Check sheet for the modelled part. Datum: model origin and axes. Units: mm. A direction names the side the tool comes from. Give positions to 0.01 mm unless a question says otherwise; leave off trailing zeros. Write each loop counter-clockwise with the first axis right and the second up, starting at its lowest first coordinate (ties: lowest second). Pieces come first, ordered by that corner, then holes. Notation, with made-up numbers: M -37.75,52.25 L -6.75,52.25 A25 ccw -6.75,83.25 Z; hole C 20.25,58.25 d3. An arc over 180 degrees is marked long. Write item = value, one per line. Start each with the question number.
1) Cross-section at A-A, the plane z = 12.5. Record the cut outline in (x, y).
2) Go/stop test with a flat-tipped pin: pin 1 (4 mm diameter, centred on x = -49.5, y = 2, fed in from +Z). Record where the tip stops, or that it passes through.
3) Mould release check, pull along Y, two halves, no side actions. Record for faces 1 (the flat face through (63.5, 5, 16)), 2 (the flat face through (-53.1, 15, 20.5)), 3 (the flat face through (-1, -25.4, 16)): released by +Y, released by -Y, zero draft, split by the parting line, or undercut.
4) Access from +Z, -Z, +X, -X, +Y, -Y to the whole of each face (thin tool, end or side, straight path). Record for faces 4 (the flat face through (23.1, -15, 20.5)), 5 (the flat face through (0, -12, 31.75)), 6 (the flat face through (0, -4.318, 20)).
5) Cross-section at D-D, the plane x = -14. Record the cut outline in (y, z), plus the area to 3 significant figures.
6) Scan lines: line 1 along X through (y, z) = (9, 11.5); line 2 along Y through (x, z) = (25, 30.5); line 3 along Y through (x, z) = (-55.5, 22). Record each from-to range of solid material in increasing order. Write a range as [from, to].
7) Cross-section at C-C, the plane y = 1.5. Record the cut outline in (x, z).
8) Cross-section at B-B, the plane x = -32. Record the cut outline in (y, z), plus the area to 3 significant figures.
```python
from build123d import *

# Parameters (mm, degrees)
BOSS_EXTRUDE1_DEPTH = 31.75
CUT_EXTRUDE1_DEPTH  = 22.86


with BuildPart() as part:
    # Sketch1 → Boss-Extrude1 (new body)
    with BuildSketch(Plane.XY):
        Polygon((63.5, -4.318), (33.782, -4.318), (12.7, -25.4), (63.5, -25.4), align=None)
        Polygon((9.467107796, -25.4), (30.549107796, -4.318), (-30.549107796, -4.318), (-9.467107796, -25.4), align=None)
        Polygon((-12.7, -25.4), (-33.782, -4.318), (-63.5, -4.318), (-63.5, -25.4), align=None)
        Polygon((12.7, -25.4), (33.782, -4.318), (30.549107796, -4.318), (9.467107796, -25.4), align=None)
        Polygon((-9.467107796, -25.4), (-30.549107796, -4.318), (-33.782, -4.318), (-12.7, -25.4), align=None)
        Polygon((39.185107796, 4.318), (60.267107796, 25.4), (-60.267107796, 25.4), (-39.185107796, 4.318), align=None)
        Polygon((30.549107796, -4.318), (39.185107796, 4.318), (-39.185107796, 4.318), (-30.549107796, -4.318), align=None)
        Polygon((63.5, 4.318), (63.5, 25.4), (42.418, 4.318), align=None)
        Polygon((63.5, 4.318), (42.418, 4.318), (33.782, -4.318), (63.5, -4.318), align=None)
        Polygon((33.782, -4.318), (42.418, 4.318), (39.185107796, 4.318), (30.549107796, -4.318), align=None)
        Polygon((42.418, 4.318), (63.5, 25.4), (60.267107796, 25.4), (39.185107796, 4.318), align=None)
        Polygon((-42.418, 4.318), (-63.5, 25.4), (-63.5, 4.318), align=None)
        Polygon((-39.185107796, 4.318), (-60.267107796, 25.4), (-63.5, 25.4), (-42.418, 4.318), align=None)
        Polygon((-33.782, -4.318), (-42.418, 4.318), (-63.5, 4.318), (-63.5, -4.318), align=None)
        Polygon((-30.549107796, -4.318), (-39.185107796, 4.318), (-42.418, 4.318), (-33.782, -4.318), align=None)
    extrude(amount=BOSS_EXTRUDE1_DEPTH)

    # Sketch2 → Cut-Extrude1 (cut)
    with BuildSketch(Plane.XY.offset(31.75)):
        Polygon((63.5, 25.4), (60.267107796, 25.4), (39.185107796, 4.318), (42.418, 4.318), align=None)
        Polygon((42.418, 4.318), (39.185107796, 4.318), (30.549107796, -4.318), (33.782, -4.318), align=None)
        Polygon((33.782, -4.318), (30.549107796, -4.318), (9.467107796, -25.4), (12.7, -25.4), align=None)
        Polygon((30.549107796, -4.318), (39.185107796, 4.318), (-39.185107796, 4.318), (-30.549107796, -4.318), align=None)
        Polygon((63.5, 4.318), (42.418, 4.318), (33.782, -4.318), (63.5, -4.318), align=None)
        Polygon((-9.467107796, -25.4), (-30.549107796, -4.318), (-33.782, -4.318), (-12.7, -25.4), align=None)
        Polygon((-30.549107796, -4.318), (-39.185107796, 4.318), (-42.418, 4.318), (-33.782, -4.318), align=None)
        Polygon((-39.185107796, 4.318), (-60.267107796, 25.4), (-63.5, 25.4), (-42.418, 4.318), align=None)
        Polygon((-33.782, -4.318), (-42.418, 4.318), (-63.5, 4.318), (-63.5, -4.318), align=None)
    extrude(amount=-CUT_EXTRUDE1_DEPTH, mode=Mode.SUBTRACT)


solid = part.part
```
Reply:
q1.outline = M -63.5,-25.4 L -12.7,-25.4 L -33.78,-4.32 L -63.5,-4.32 Z; M -63.5,4.32 L -42.42,4.32 L -63.5,25.4 Z; M -60.27,25.4 L -39.19,4.32 L 39.19,4.32 L 60.27,25.4 Z; M -30.55,-4.32 L -9.47,-25.4 L 9.47,-25.4 L 30.55,-4.32 Z; M 12.7,-25.4 L 63.5,-25.4 L 63.5,-4.32 L 33.78,-4.32 Z; M 42.42,4.32 L 63.5,4.32 L 63.5,25.4 Z
q2.pin_1 = 8.89
q3.face_1 = zero draft
q3.face_2 = undercut
q3.face_3 = released by -Y
q4.face_4 = +Z
q4.face_5 = +Z, +X, -X, +Y, -Y
q4.face_6 = +Z, +X, -X
q5.outline = M -25.4,0 L 25.4,0 L 25.4,31.75 L 4.32,31.75 L 4.32,8.89 L -4.32,8.89 L -4.32,31.75 L -20.87,31.75 L -20.87,8.89 L -24.1,8.89 L -24.1,31.75 L -25.4,31.75 Z
q5.area = 1,340 mm2
q6.line_1 = [-63.5, -47.1], [-43.87, 43.87], [47.1, 63.5]
q6.line_2 = [-25.4, -13.1], [-9.87, -4.32], [4.32, 25.4]
q6.line_3 = [-25.4, -4.32], [4.32, 17.4], [20.63, 25.4]
q7.outline = M -63.5,0 L 63.5,0 L 63.5,8.89 L -63.5,8.89 Z
q8.outline = M -25.4,0 L 25.4,0 L 25.4,31.75 L 4.32,31.75 L 4.32,8.89 L -6.1,8.89 L -6.1,31.75 L -25.4,31.75 Z
q8.area = 1,370 mm2
